```python
from build123d import *

# Parameters (mm, degrees)
EXTRUDE_1_DEPTH             = 50
SKETCH_2_R                  = 2
EXTRUDE_2_DEPTH             = 6
SKETCH_3_R                  = 2
SKETCH_3_R_2                = 1.6
CUT_EXTRUDE_3_DEPTH         = 0.5
CHAMFER_1_SIZE              = 0.4
HOLE_WIZARD_M31_D           = 2.2
HOLE_WIZARD_M31_DEPTH       = 8
HOLE_WIZARD_M31_CSINK_D     = 3
HOLE_WIZARD_M31_CSINK_ANGLE = 90
HOLE_WIZARD_M31_TIP         = 0.660946681


with BuildPart() as part:
    # Эскиз1 → Вытянуть1 (new body)
    with BuildSketch(Plane.XY):
        Polygon((0, 4.041451884), (-3.5, 2.020725942), (-3.5, -2.020725942), (0, -4.041451884), (3.5, -2.020725942), (3.5, 2.020725942), align=None)
    extrude(amount=EXTRUDE_1_DEPTH)

    # Эскиз2 → Вытянуть2 (add)
    with BuildSketch(Plane.XY.offset(50)):
        Circle(SKETCH_2_R)
    extrude(amount=EXTRUDE_2_DEPTH)

    # Эскиз3 → Вырез-Вытянуть3 (cut)
    with BuildSketch(Plane.XY.offset(50)):
        Circle(SKETCH_3_R)
        Circle(SKETCH_3_R_2, mode=Mode.SUBTRACT)
    extrude(amount=CUT_EXTRUDE_3_DEPTH, mode=Mode.SUBTRACT)

    # Фаска1
    chamfer_1_edges = [part.edges().sort_by_distance(p)[0] for p in [
        (-2, 0, 56),
        (-2, 0, 50.5),
    ]]
    chamfer(chamfer_1_edges, length=CHAMFER_1_SIZE - 0.0001)  # a hair under: the kernel refuses the full size

    # Отверстие с зазором M31
    with Locations(Plane(origin=(0, 0, 0), x_dir=(-1, 0, 0), z_dir=(0, 0, -1))):
        with Locations((0, 0)):
            CounterSinkHole(HOLE_WIZARD_M31_D / 2, HOLE_WIZARD_M31_CSINK_D / 2, depth=HOLE_WIZARD_M31_DEPTH, counter_sink_angle=HOLE_WIZARD_M31_CSINK_ANGLE)
            with Locations((0, 0, -(HOLE_WIZARD_M31_DEPTH + HOLE_WIZARD_M31_TIP / 2))):  # 118° drill point
                Cone(0, HOLE_WIZARD_M31_D / 2, HOLE_WIZARD_M31_TIP, mode=Mode.SUBTRACT)


solid = part.part
```
Geometry check sheet. Reference: the model listing, model coordinates, mm. A direction names the side the tool comes from. Give positions to 0.01 mm unless a question says otherwise; leave off trailing zeros. Order: outer loops, then holes, each group sorted by start corner. A loop starts at its lowest first (then second) coordinate and runs counter-clockwise, first axis right, second up. Notation, with made-up numbers: (40, -7.5) -> (76, -7.5) arc R34 cw to (76, 30.5) -> close; hole circle Ø4 at (86.25, 16.25). An arc over 180 degrees is marked (long way). Write each question's results on one line, items separated by ' | '. Start each with the question number.
(1) Gauge pin test, flat ends, axial feed: P1, Ø1.6, axis at x = 0, y = 0.5, coming from the -Z side; P2, Ø1.5, axis at x = 2.5, z = 15.5, coming from the -Y side. Record the tip position at first contact, or that the pin passes through.
(2) Sectioned sample at A-A (z = 17.5). Enter the section's corners in (x, y), plus the area to 3 significant figures.
(3) Mould release check, pull along Y, two halves, no side actions. Record for faces 1 (the face through (0.041, -0.186, 8.546)), 2 (the face through (0, -2, 0)), 3 (the face through (0, -2, 53)), 4 (the face through (1.05, 0.33, 4.25)): pulls with the +Y half, pulls with the -Y half, needs draft (parallel to the pull), parting line crosses it, or undercut.
(4) Sectioned sample at C-C (z = 52). Enter the section's corners in (x, y).
(5) Scan lines: line 1 (X direction, y = 0, z = 5.25); line 2 (Y direction, x = 0, z = 5.75); line 3 (Z direction, x = 0.5, y = -2.75). Record each from-to range of solid material in increasing order.
(6) Access from +Z, -Z, +X, -X, +Y, -Y to the whole of each face (thin tool, end or side, straight path). Record for faces 5 (the face through (1.726, -3.045, 24.65)), 6 (the face through (-1.27, -0.97, 50.25)).
(7) Sectioned sample at B-B (x = 2.75). Enter the section's corners in (y, z), plus the area to 3 significant figures.
Answer below:
1) P1: z = 0.2 | P2: y = -3.03
2) outline: (-3.5, -2.02) -> (0, -4.04) -> (3.5, -2.02) -> (3.5, 2.02) -> (0, 4.04) -> (-3.5, 2.02) -> close | area: 42.4 mm2
3) face 1: undercut | face 2: needs draft | face 3: parting line crosses it | face 4: undercut
4) outline: circle Ø4 at (0, 0)
5) line 1: -3.5 to -1.1, 1.1 to 3.5 | line 2: -4.04 to -1.1, 1.1 to 4.04 | line 3: 0 to 50
6) face 5: +Z, -Z, +X, -Y | face 6: none
7) outline: (-2.45, 0) -> (2.45, 0) -> (2.45, 50) -> (-2.45, 50) -> close | area: 245 mm2
